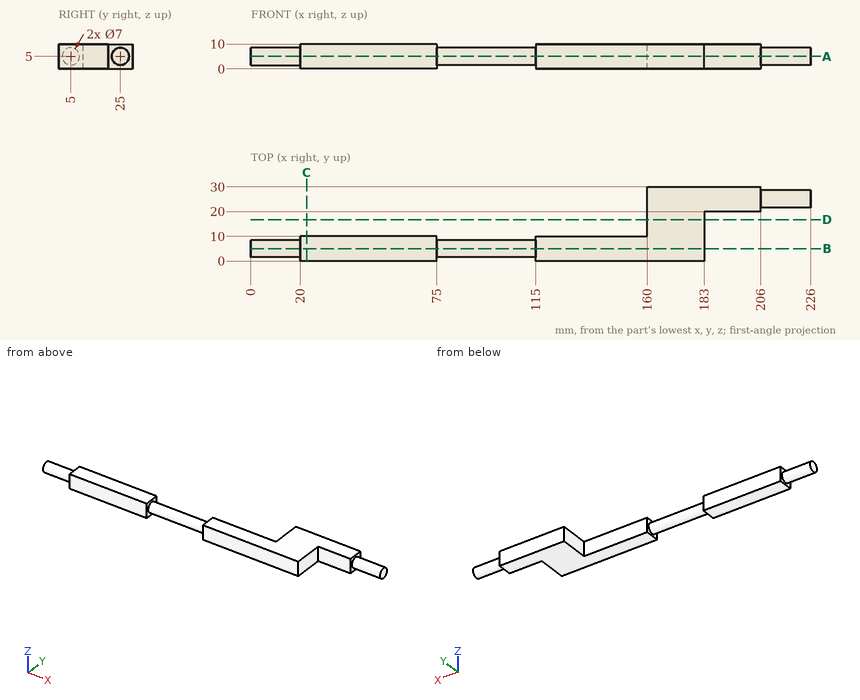
Design review of the part shown in the three views and the two pictorial views. Dimensions are in mm from the part's minimum x, y and z. Round coordinates to 2 decimals unless told otherwise and drop trailing zeros. Loops run counter-clockwise (first coordinate to the right, second up) from the corner with the lowest first, then second, coordinate; pieces in that order, holes last. Notation, with made-up numbers: (78, 56) -> (112, 56) arc R24 cw to (112, 69) -> close; hole circle Ø4 at (-27.75, -3). An arc over 180 degrees is marked (long way). Answer as CSV lines item,"result".
1) For P1, Ø5, axis at x = 38, z = 5.5, coming from the +Y side; P2, Ø1, axis at x = 86.5, z = 6.5, coming from the +Y side; P3, Ø5, axis at y = 22.5, z = 4, coming from the -X side, all flat-tipped, find the tip position at first contact; note any pin that passes through.
Geometry results:
P1,"stops at y = 10"
P2,"stops at y = 8.35"
P3,"stops at x = 160"
2) Add section A-A on z = 5. Write out the cut boundary in (x, y).
Geometry results:
outline,"(0, 1.5) -> (20, 1.5) -> (20, 0) -> (75, 0) -> (75, 1.5) -> (115, 1.5) -> (115, 0) -> (183, 0) -> (183, 20) -> (206, 20) -> (206, 21.5) -> (226, 21.5) -> (226, 28.5) -> (206, 28.5) -> (206, 30) -> (160, 30) -> (160, 10) -> (115, 10) -> (115, 8.5) -> (75, 8.5) -> (75, 10) -> (20, 10) -> (20, 8.5) -> (0, 8.5) -> close"
3) Add section C-C on x = 22.5. Write out the cut boundary in (y, z).
Geometry results:
outline,"(0, 0) -> (10, 0) -> (10, 10) -> (0, 10) -> close"
4) Add section B-B on y = 5. Write out the cut boundary in (x, z), plus the area to 3 significant figures.
Geometry results:
outline,"(0, 1.5) -> (20, 1.5) -> (20, 0) -> (75, 0) -> (75, 1.5) -> (115, 1.5) -> (115, 0) -> (183, 0) -> (183, 10) -> (115, 10) -> (115, 8.5) -> (75, 8.5) -> (75, 10) -> (20, 10) -> (20, 8.5) -> (0, 8.5) -> close"
area,"1,650 mm²"
5) Add section D-D on y = 16.75. Write out the cut boundary in (x, z).
Geometry results:
outline,"(160, 0) -> (183, 0) -> (183, 10) -> (160, 10) -> close"
6) To check wall thickness, follow line 1 along X through (y, z) = (8.75, 9); line 2 along X through (y, z) = (2, 5.75); line 3 along X through (y, z) = (28.75, 3). State the ranges of each line that lie inside material, in increasing order. Write a range as from..to.
Geometry results:
line 1,"x = 20..75, 115..183"
line 2,"x = 0..183"
line 3,"x = 160..206"
